Read the model definition and answer for the solid it produces. Units are mm, in the model's axes. Face numbers are marked on the shaded views. A direction names the side the tool comes from. Coordinates: 2 decimals unless noted, no trailing zeros. Write each loop counter-clockwise with the first axis right and the second up, starting at its lowest first coordinate (ties: lowest second). Pieces come first, ordered by that corner, then holes. Notation, with made-up numbers: (30.5, 87.25) - (48.5, 87.25) arc R24 cw to (48.5, 113.25) - close; hole circle Ø6 at (16, 71). An arc over 180 degrees is marked (long way). Return JSON: item names as keys, results as strings.
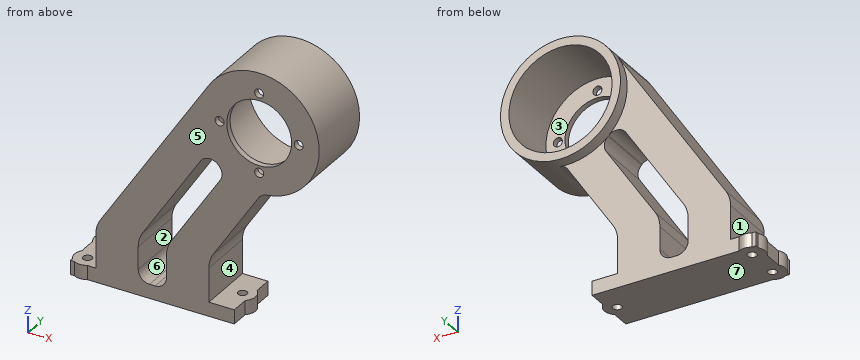
```python
from build123d import *

# Parameters (mm, degrees)
SKETCH1_R           = 18.25
SKETCH1_R_2         = 1.6
SKETCH1_R_3         = 11.5
BOSS_EXTRUDE1_DEPTH = 2
SKETCH1_3_R         = 21.25
SKETCH1_3_R_2       = 18.25
BOSS_EXTRUDE2_DEPTH = 24
BOSS_EXTRUDE3_DEPTH = 20
SKETCH3_R           = 1.6
BOSS_EXTRUDE4_DEPTH = 5
FILLET3_R           = 10
FILLET4_R           = 4


with BuildPart() as part:
    # Sketch1 → Boss-Extrude1 (new body)
    with BuildSketch(Plane(origin=(0, 0, 0), x_dir=(1, 0, 0), z_dir=(0, 1, 0))):
        Circle(SKETCH1_R)
        with Locations((-14, 0)):
            Circle(SKETCH1_R_2, mode=Mode.SUBTRACT)
        with Locations((0, -14)):
            Circle(SKETCH1_R_2, mode=Mode.SUBTRACT)
        with Locations((14, 0)):
            Circle(SKETCH1_R_2, mode=Mode.SUBTRACT)
        with Locations((0, 14)):
            Circle(SKETCH1_R_2, mode=Mode.SUBTRACT)
        Circle(SKETCH1_R_3, mode=Mode.SUBTRACT)
    extrude(amount=BOSS_EXTRUDE1_DEPTH)

    # Sketch1<3> → Boss-Extrude2 (add)
    with BuildSketch(Plane(origin=(0, 0, 0), x_dir=(1, 0, 0), z_dir=(0, 1, 0))):
        Circle(SKETCH1_3_R)
        Circle(SKETCH1_3_R_2, mode=Mode.SUBTRACT)
    extrude(amount=BOSS_EXTRUDE2_DEPTH)

    # Sketch2 → Boss-Extrude3 (add)
    with BuildSketch(Plane(origin=(0, 0, 0), x_dir=(1, 0, 0), z_dir=(0, 1, 0))):
        with BuildLine():
            ThreePointArc((-17.839967658, -11.545477642), (-21.249992199, 0.018208346), (-17.820155675, 11.576033506))
            Line((-17.820155675, 11.576033506), (-57.820155675, -50))
            Line((-57.820155675, -50), (-57.820155675, -70))
            Line((-57.820155675, -70), (-42.820155675, -70))
            Line((-42.820155675, -70), (-42.820155675, -50))
            Line((-42.820155675, -50), (-17.839967658, -11.545477642))
        make_face()
        with BuildLine():
            Line((-17.820155675, -50), (0.867447809, -21.232287543))
            ThreePointArc((0.867447809, -21.232287543), (-5.756886716, -20.45533562), (-11.81408432, -17.663236161))
            Line((-11.81408432, -17.663236161), (-32.820155675, -50))
            Line((-32.820155675, -50), (-32.820155675, -70))
            Line((-32.820155675, -70), (-17.820155675, -70))
            Line((-17.820155675, -70), (-17.820155675, -50))
        make_face()
    extrude(amount=BOSS_EXTRUDE3_DEPTH)

    # Sketch3 → Boss-Extrude4 (add)
    with BuildSketch(Plane.XY.offset(70)):
        with BuildLine():
            Line((-65.389940295, 20), (-66.820155675, 20))
            Line((-66.820155675, 20), (-66.820155675, 18.730720476))
            ThreePointArc((-66.820155675, 18.730720476), (-67.718376956, 16), (-66.820155675, 13.269279524))
            Line((-66.820155675, 13.269279524), (-66.820155675, 6.730720476))
            ThreePointArc((-66.820155675, 6.730720476), (-67.718376956, 4), (-66.820155675, 1.269279524))
            Line((-66.820155675, 1.269279524), (-66.820155675, 0))
            Line((-66.820155675, 0), (-65.389940295, 0))
            ThreePointArc((-65.389940295, 0), (-63.118376956, -0.6), (-60.846813618, 0))
            Line((-60.846813618, 0), (-8.820155675, 0))
            Line((-8.820155675, 0), (-8.820155675, 6.512880845))
            ThreePointArc((-8.820155675, 6.512880845), (-7.220155675, 10), (-8.820155675, 13.487119155))
            Line((-8.820155675, 13.487119155), (-8.820155675, 20))
            Line((-8.820155675, 20), (-60.846813618, 20))
            ThreePointArc((-60.846813618, 20), (-63.118376956, 20.6), (-65.389940295, 20))
        make_face()
        with Locations((-63.118376956, 16)):
            Circle(SKETCH3_R, mode=Mode.SUBTRACT)
        with Locations((-63.118376956, 4)):
            Circle(SKETCH3_R, mode=Mode.SUBTRACT)
        with Locations((-11.820155675, 10)):
            Circle(SKETCH3_R, mode=Mode.SUBTRACT)
    extrude(amount=-BOSS_EXTRUDE4_DEPTH)

    # Fillet3
    fillet3_edges = [part.edges().sort_by_distance(p)[0] for p in [
        (-57.820155675, 10, 50),
        (-42.820155675, 10, 50),
        (-32.820155675, 10, 50),
        (-17.820155675, 10, 50),
    ]]
    fillet(fillet3_edges, radius=FILLET3_R)

    # Fillet4
    fillet4_edges = [part.edges().sort_by_distance(p)[0] for p in [
        (-17.839967658, 10, 11.545477642),
        (0.867447809, 10, 21.232287543),
        (-11.81408432, 10, 17.663236161),
        (-42.820155675, 10, 65),
        (-32.820155675, 10, 65),
    ]]
    fillet(fillet4_edges, radius=FILLET4_R)


with BuildPart() as body_2:
    # Mirror1: mirrored copy
    add(part.part.mirror(Plane(origin=(0, 20, 70), x_dir=(1, 0, 0), z_dir=(0, 0, -1))))


solid = body_2.part
```
(1) Determine the mould class of the marked faces 5, 6 and 7 for opening direction Z: +Z half, -Z half, draft (parallel to the pull), parting line (faces both ways), or undercut.
Answer:
{"face 5": "draft", "face 6": "undercut", "face 7": "-Z half"}
(2) A cutting plane is placed at C-C (x = 14). Determine the outline of the cut face in (y, z).
Answer:
{"outline": "(0, 124.01) - (24, 124.01) - (24, 128.29) - (2, 128.29) - (2, 138.4) - (0, 138.4) - close; (0, 141.6) - (2, 141.6) - (2, 151.71) - (24, 151.71) - (24, 155.99) - (0, 155.99) - close"}
(3) Straight lines are drawn through the part: line 1 (Z direction, x = 0, y = 0.6); line 2 (Z direction, x = -14, y = 0.8); line 3 (Z direction, x = -8.5, y = 9). For each, find the intervals that lie inside material, in ascending order. Write a range as from..to.
Answer:
{"line 1": "117.41..124.4, 127.6..128.5, 151.5..152.4, 155.6..161.25", "line 2": "70..75, 95.88..118.97, 123.93..138.4, 141.6..155.99", "line 3": "70..75, 104.35..123.85, 156.15..159.48"}
(4) Flat-ended cylindrical pins translate along their axes: P1, Ø12, axis at y = 5, z = 132, coming from the -X side; P2, Ø5, axis at x = -18, y = 5, coming from the +Z side; P3, Ø2.5, axis at y = 11, z = 73.5, coming from the -X side; P4, Ø2.5, axis at x = -63.12, y = 16, coming from the -Z side. Find the tip coordinate at first contact, or state that the pin passes through.
Answer:
{"P1": "x = -34.43", "P2": "z = 154.54", "P3": "x = -66.82", "P4": "through"}
(5) A cutting plane is placed at B-B (z = 111.5). Determine the outline of the cut face in (x, y).
Answer:
{"outline": "(-43.85, 0) - (-28.85, 0) - (-28.85, 20) - (-43.85, 20) - close; (-18.85, 0) - (-3.85, 0) - (-3.85, 20) - (-18.85, 20) - close"}
(6) A cutting plane is placed at A-A (y = 10). State how many separate pieces and enclosed holes the cut face has, and give its area (3 significant figures).
Answer:
{"separate pieces": "2", "enclosed holes": "2", "area": "2,270 mm²"}
(7) Which of the six approach directions +Z, -Z, +X, -X, +Y, -Y give full straight-line access (tool end or side, diameter ignored) to the marked faces 1, 2, 3 and 4?
Answer:
{"face 1": "+Z, -X, +Y, -Y", "face 2": "+Y, -Y", "face 3": "+Y", "face 4": "+X, +Y, -Y"}
